Could you check a few things on this drawing? It's one solid part, dimensions in mm from its lowest x, y, z. A direction names the side the tool comes from. Round coordinates to 2 decimals unless told otherwise and drop trailing zeros. Loops run counter-clockwise (first coordinate to the right, second up) from the corner with the lowest first, then second, coordinate; pieces in that order, holes last. Notation, with made-up numbers: (40, -1.75) -> (76, -1.75) arc R24 ccw to (76, 36.25) -> close; hole circle Ø2 at (8.25, 4). An arc over 180 degrees is marked (long way). Put each result on its own line as item: value. Start each with the question number.
1. Imagine slicing it at D-D, the plane z = 3. Please give me the cut outline in (x, y) (1 decimal).
2. Imagine slicing it at C-C, the plane x = 20. Please give me the cut outline in (y, z).
3. Imagine slicing it at B-B, the plane y = 0.4. Count the separate pieces of the cut face and the enclosed holes in it.
4. Imagine slicing it at A-A, the plane z = 15. Please give me the cut outline in (x, y).
5. I'm going to push flat-ended pins straight in: P1, Ø1.5, axis at x = 24.5, y = 2, coming from the +Z side; P2, Ø10, axis at x = 12.5, z = 5, coming from the +Y side; P3, Ø2, axis at y = 2, z = 4.5, coming from the -X side. Where does each tip first touch, or does it pass through?
6. Which directions (+Z, -Z, +X, -X, +Y, -Y) give clear straight access to the entire face, cutting with the end or side of a thin tool? Please do the marked faces 1 and 2.
7. If we mould it in two halves opening along Z, with no side actions, what happens to the marked faces 3, 4, 5 and 6? For each: pulls with the +Z half, pulls with the -Z half, needs draft (parallel to the pull), parting line crosses it, or undercut.
8. I need wall thicknesses on line 1 (Z direction, x = 13.5, y = 0.45); line 2 (X direction, y = 1.15, z = 13.5). Which ranges of each line are inside material? Lowest first, please. Write a range as [from, to].
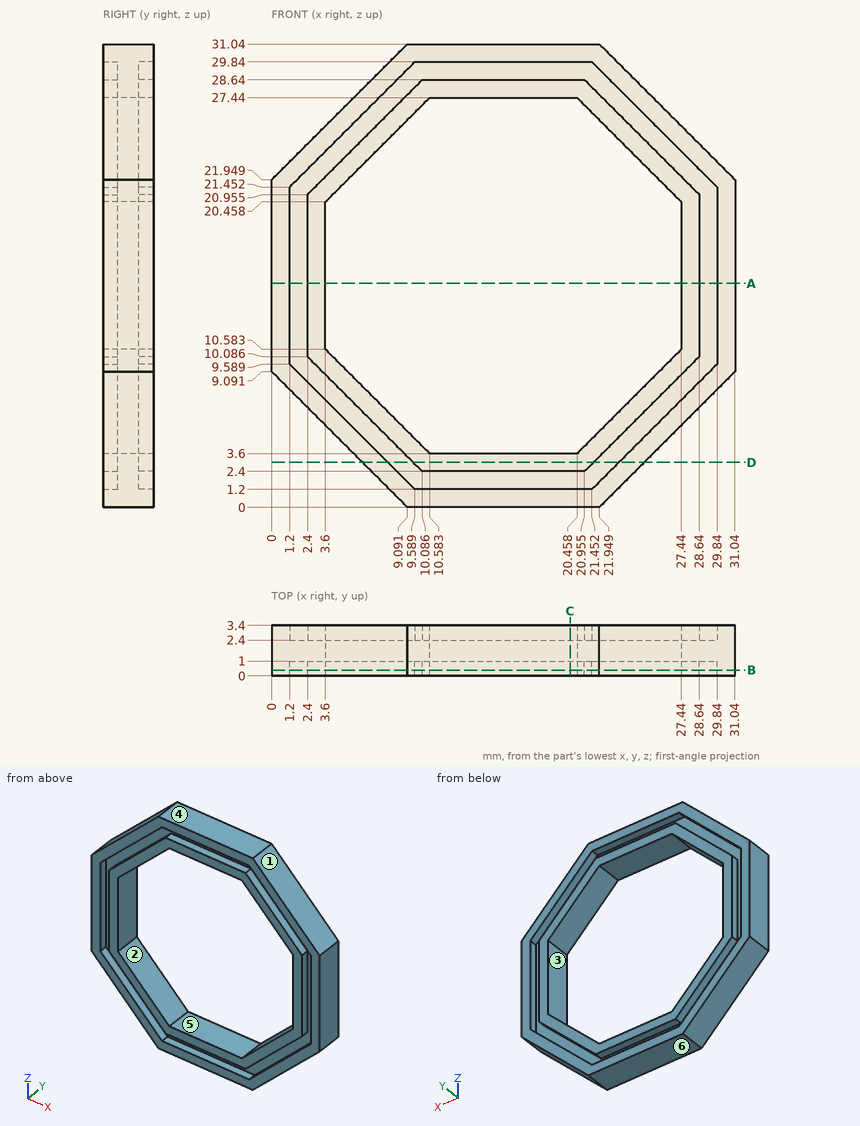
Entries:
1. outline: (6.1, 0) -> (7.8, 0) -> (7.8, 1) -> (9.5, 1) -> (9.5, 0) -> (21.6, 0) -> (21.6, 1) -> (23.3, 1) -> (23.3, 0) -> (24.9, 0) -> (24.9, 3.4) -> (23.3, 3.4) -> (23.3, 2.4) -> (21.6, 2.4) -> (21.6, 3.4) -> (9.5, 3.4) -> (9.5, 2.4) -> (7.8, 2.4) -> (7.8, 3.4) -> (6.1, 3.4) -> close
2. outline: (0, 0) -> (3.4, 0) -> (3.4, 1.2) -> (2.4, 1.2) -> (2.4, 2.4) -> (3.4, 2.4) -> (3.4, 3.6) -> (0, 3.6) -> (0, 2.4) -> (1, 2.4) -> (1, 1.2) -> (0, 1.2) -> close; (0, 27.44) -> (3.4, 27.44) -> (3.4, 28.64) -> (2.4, 28.64) -> (2.4, 29.84) -> (3.4, 29.84) -> (3.4, 31.04) -> (0, 31.04) -> (0, 29.84) -> (1, 29.84) -> (1, 28.64) -> (0, 28.64) -> close
3. separate pieces: 2
3. enclosed holes: 2
4. outline: (0, 0) -> (1.2, 0) -> (1.2, 1) -> (2.4, 1) -> (2.4, 0) -> (3.6, 0) -> (3.6, 3.4) -> (2.4, 3.4) -> (2.4, 2.4) -> (1.2, 2.4) -> (1.2, 3.4) -> (0, 3.4) -> close; (27.44, 0) -> (28.64, 0) -> (28.64, 1) -> (29.84, 1) -> (29.84, 0) -> (31.04, 0) -> (31.04, 3.4) -> (29.84, 3.4) -> (29.84, 2.4) -> (28.64, 2.4) -> (28.64, 3.4) -> (27.44, 3.4) -> close
5. P1: z = 29.24
5. P2: y = 3.4
5. P3: x = 3.59
6. face 1: +Z, +X, +Y, -Y
6. face 2: +Y, -Y
7. face 3: undercut
7. face 4: pulls with the +Z half
7. face 5: undercut
7. face 6: pulls with the -Z half
8. line 1: [0, 1.2], [2.4, 3.6], [27.44, 28.64], [29.84, 31.04]
8. line 2: [0, 3.6], [27.44, 31.04]
